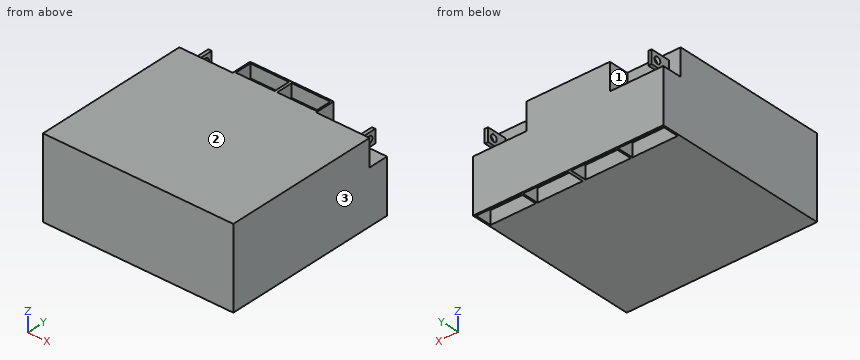
Autodesk Inventor part; units mm, degrees
ref_plane "YZ Plane" through (0, 0, 0) normal (1, 0, 0) x (0, 1, 0)
ref_plane "XZ Plane" through (0, 0, 0) normal (0, 1, 0) x (-1, 0, 0)
ref_plane "XY Plane" through (0, 0, 0) normal (0, 0, 1) x (1, 0, 0)
sketch "Sketch1" plane through (0, 0, 0) normal (0, 1, 0) x (-1, 0, 0)
  line L0 (0, 0) -> (-180.975, 0)
  line L1 (-180.975, 0) -> (-180.975, -76.2)
  line L2 (-180.975, -76.2) -> (0, -76.2)
  line L3 (0, -76.2) -> (0, 0)
  dimension "d0" = 180.975
  dimension "d1" = 76.2
extrude "Extrusion1" add sketch "Sketch1" along normal blind 168.275
sketch "Sketch2" plane through (0, 168.275, 0) normal (0, 1, 0) x (1, 0, 0)
  line L0 (0, 0) -> (180.975, 0)
  line L1 (180.975, 0) -> (180.975, 76.2)
  line L2 (180.975, 76.2) -> (0, 76.2)
  line L3 (0, 76.2) -> (0, 0)
  line L4 (0, 0) -> (50.8, 0)
  line L5 (50.8, 0) -> (50.8, 25.4)
  line L6 (50.8, 25.4) -> (0, 25.4)
  line L7 (0, 25.4) -> (0, 0)
  line L8 (180.975, 0) -> (130.175, 0)
  line L9 (130.175, 0) -> (130.175, 25.4)
  line L10 (130.175, 25.4) -> (180.975, 25.4)
  line L11 (180.975, 25.4) -> (180.975, 0)
  dimension "d4" = 50.8
  dimension "d5" = 25.4
  dimension "d6" = 50.8
  dimension "d7" = 25.4
extrude "Extrusion2" cut sketch "Sketch2" against normal blind 19.05 contours L3 L6 L5 L0 | L9 L10 L1 L0
sketch "Sketch3" plane through (0, 0, 0) normal (0, 0, 1) x (1, 0, 0)
  line L0 (50.8, 168.275) -> (50.8, 149.225) construction
  line L1 (50.8, 149.225) -> (0, 149.225)
  line L2 (0, 0) -> (0, 149.225)
  line L3 (0, 0) -> (180.975, 0)
  line L4 (180.975, 0) -> (180.975, 149.225)
  line L5 (180.975, 149.225) -> (130.175, 149.225)
  line L6 (130.175, 149.225) -> (130.175, 168.275) construction
  line L7 (50.8, 168.275) -> (130.175, 168.275) construction
  line L8 (50.8, 168.275) -> (130.175, 168.275)
  line L9 (130.175, 168.275) -> (130.175, 149.225)
  line L10 (130.175, 149.225) -> (50.8, 149.225) construction
  line L11 (50.8, 149.225) -> (50.8, 168.275)
  line L12 (52.3875, 150.8125) -> (128.5875, 150.8125) construction
  line L13 (128.5875, 150.8125) -> (128.5875, 166.6875) construction
  line L14 (128.5875, 166.6875) -> (52.3875, 166.6875) construction
  line L15 (52.3875, 166.6875) -> (52.3875, 150.8125) construction
  line L16 (52.3875, 166.6875) -> (89.2175, 166.6875)
  line L17 (89.2175, 166.6875) -> (89.2175, 150.8125)
  line L18 (89.2175, 150.8125) -> (52.3875, 150.8125)
  line L19 (52.3875, 150.8125) -> (52.3875, 166.6875)
  line L20 (128.5875, 150.8125) -> (91.7575, 150.8125)
  line L21 (91.7575, 150.8125) -> (91.7575, 166.6875)
  line L22 (91.7575, 166.6875) -> (128.5875, 166.6875)
  line L23 (128.5875, 166.6875) -> (128.5875, 150.8125)
  dimension "d10" = 1.5875
  dimension "d11" = 36.83
  dimension "d12" = 36.83
extrude "Extrusion3" cut sketch "Sketch3" against normal blind 12.7 contours L16 L17 L18 L19 | L20 L21 L22 L23
sketch "Sketch4" plane through (180.975, 0, -76.2) normal (0, 0, -1) x (-1, 0, 0)
  line L0 (0, 0) -> (180.975, 0) construction
  line L1 (180.975, 0) -> (180.975, 168.275) construction
  line L2 (0, 168.275) -> (180.975, 168.275) construction
  line L3 (0, 0) -> (0, 168.275) construction
  line L4 (0, 168.275) -> (180.975, 168.275) construction
  line L5 (180.975, 168.275) -> (180.975, 149.225) construction
  line L6 (180.975, 149.225) -> (0, 149.225) construction
  line L7 (0, 149.225) -> (0, 168.275) construction
  line L8 (1.5875, 150.8125) -> (179.3875, 150.8125) construction
  line L9 (179.3875, 150.8125) -> (179.3875, 166.6875) construction
  line L10 (179.3875, 166.6875) -> (1.5875, 166.6875) construction
  line L11 (1.5875, 166.6875) -> (1.5875, 150.8125) construction
  line L12 (1.5875, 166.6875) -> (44.5135, 166.6875)
  line L13 (44.5135, 166.6875) -> (44.5135, 150.8125)
  line L14 (44.5135, 150.8125) -> (1.5875, 150.8125)
  line L15 (1.5875, 150.8125) -> (1.5875, 166.6875)
  line L16 (179.3875, 150.8125) -> (136.4615, 150.8125)
  line L17 (136.4615, 150.8125) -> (136.4615, 166.6875)
  line L18 (136.4615, 166.6875) -> (179.3875, 166.6875)
  line L19 (179.3875, 166.6875) -> (179.3875, 150.8125)
  line L20 (46.101, 150.8125) -> (89.027, 150.8125)
  line L21 (89.027, 150.8125) -> (89.027, 166.6875)
  line L22 (89.027, 166.6875) -> (46.101, 166.6875)
  line L23 (46.101, 166.6875) -> (46.101, 150.8125)
  line L24 (134.874, 150.8125) -> (91.948, 150.8125)
  line L25 (91.948, 150.8125) -> (91.948, 166.6875)
  line L26 (91.948, 166.6875) -> (134.874, 166.6875)
  line L27 (134.874, 166.6875) -> (134.874, 150.8125)
  dimension "d15" = 1.5875
  dimension "d16" = 42.926
  dimension "d17" = 42.926
  dimension "d18" = 42.926
  dimension "d19" = 42.926
  dimension "d20" = 1.5875
  dimension "d21" = 1.5875
extrude "Extrusion4" cut sketch "Sketch4" against normal blind 12.7
sketch "Sketch5" plane through (0, 149.225, 0) normal (0, 1, 0) x (1, 0, 0)
  line L0 (50.8, 0) -> (0, 0)
  line L1 (50.8, 25.4) -> (50.8, 0)
  line L2 (0, 25.4) -> (50.8, 25.4)
  line L3 (0, 0) -> (0, 25.4)
  line L4 (180.975, 25.4) -> (180.975, 0)
  line L5 (130.175, 25.4) -> (180.975, 25.4)
  line L6 (130.175, 0) -> (130.175, 25.4)
  line L7 (180.975, 0) -> (130.175, 0)
  line L8 (0, 0) -> (12.7, 0) construction
  line L9 (12.7, 0) -> (12.7, 12.7) construction
  line L10 (12.7, 12.7) -> (0, 12.7) construction
  line L11 (0, 12.7) -> (0, 0) construction
  line L12 (180.975, 0) -> (168.275, 0) construction
  line L13 (168.275, 0) -> (168.275, 12.7) construction
  line L14 (168.275, 12.7) -> (180.975, 12.7) construction
  line L15 (180.975, 12.7) -> (180.975, 0) construction
  line L16 (11.1125, 19.05) -> (14.2875, 19.05)
  line L17 (14.2875, 19.05) -> (14.2875, 6.35)
  line L18 (14.2875, 6.35) -> (11.1125, 6.35)
  line L19 (11.1125, 6.35) -> (11.1125, 19.05)
  line L20 (11.1125, 19.05) -> (14.2875, 6.35) construction
  line L21 (14.2875, 19.05) -> (11.1125, 6.35) construction
  line L22 (169.8625, 6.35) -> (166.6875, 6.35)
  line L23 (166.6875, 6.35) -> (166.6875, 19.05)
  line L24 (166.6875, 19.05) -> (169.8625, 19.05)
  line L25 (169.8625, 19.05) -> (169.8625, 6.35)
  line L26 (169.8625, 6.35) -> (166.6875, 19.05) construction
  line L27 (166.6875, 6.35) -> (169.8625, 19.05) construction
  dimension "d24" = 12.7
  dimension "d25" = 12.7
  dimension "d26" = 12.7
  dimension "d27" = 12.7
  dimension "d28" = 3.175
  dimension "d29" = 12.7
  dimension "d30" = 3.175
  dimension "d31" = 12.7
extrude "Extrusion5" add sketch "Sketch5" along normal blind 19.05 contours L16 L17 L18 L19 | L22 L23 L24 L25
sketch "Sketch6" plane through (169.8625, 149.225, -6.35) normal (1, 0, 0) x (0, 0, -1)
  line L0 (12.7, 0) -> (0, 0) construction
  line L1 (12.7, 0) -> (12.7, 19.05) construction
  line L2 (0, 19.05) -> (12.7, 19.05) construction
  line L3 (0, 0) -> (0, 19.05) construction
  line L4 (0, 19.05) -> (6.35, 19.05) construction
  line L5 (6.35, 19.05) -> (6.35, 12.7) construction
  line L6 (6.35, 12.7) -> (0, 12.7) construction
  line L7 (0, 12.7) -> (0, 19.05) construction
  circle A0 centre (6.35, 12.7) radius 3.175
  point P0 (-6.35, -149.225)
  dimension "d34" = 6.35
  dimension "d35" = 6.35
  dimension "d36" = 6.35
extrude "Extrusion6" cut sketch "Sketch6" against normal blind 25.4
sketch "Sketch7" plane through (11.1125, 149.225, -19.05) normal (-1, 0, 0) x (0, 0, 1)
  line L0 (12.7, 0) -> (0, 0) construction
  line L1 (12.7, 0) -> (12.7, 19.05) construction
  line L2 (0, 19.05) -> (12.7, 19.05) construction
  line L3 (0, 0) -> (0, 19.05) construction
  line L4 (12.7, 19.05) -> (6.35, 19.05) construction
  line L5 (6.35, 19.05) -> (6.35, 12.7) construction
  line L6 (6.35, 12.7) -> (12.7, 12.7) construction
  line L7 (12.7, 12.7) -> (12.7, 19.05) construction
  circle A0 centre (6.35, 12.7) radius 3.175
  point P0 (19.05, -149.225)
  dimension "d39" = 6.35
  dimension "d40" = 6.35
  dimension "d41" = 6.35
extrude "Extrusion7" cut sketch "Sketch7" against normal blind 25.4
properties part number "battery"
Verification items for the finished model (mm, model axes). Face numbers are marked on the shaded views. Coordinates: 2 decimals unless noted, no trailing zeros. Loops run counter-clockwise (first coordinate to the right, second up) from the corner with the lowest first, then second, coordinate; pieces in that order, holes last. Notation, with made-up numbers: (15, 15) -> (38, 15) arc R8 cw to (38, 26) -> close; hole circle Ø5 at (73.5, 58.5). An arc over 180 degrees is marked (long way). Answer as a JSON object with one key per item and string values. Group by question number.
Item 1: Mould release check, pull along X, two halves, no side actions. Record for the marked faces 1, 2 and 3: +X half, -X half, draft (parallel to the pull), parting line (faces both ways), or undercut.
Item 2: Sectioned sample at A-A on x = 56. Record the boundary of the cut face in (y, z) (1 decimal), plus the area to 3 significant figures.
Item 3: Depth check by flat-ended pin: pin 1 (5.5 mm diameter, centred on y = 158.5, z = -18.5, fed in from +X); pin 2 (9.5 mm diameter, centred on y = 163, z = -11, fed in from -X). Enter the tip coordinate at first touch or a pass-through.
Item 4: Scan lines: probe 1 along Y at (x, z) = (13.1, -12.7) (3 decimals); probe 2 along Y at (x, z) = (118.5, -73) (1 decimal); probe 3 along Y at (x, z) = (22, -19) (3 decimals). Record each from-to range of solid material in increasing order.
Evaluation:
{
 "1": {"face 1": "undercut", "face 2": "draft", "face 3": "+X half"},
 "2": {"outline": "(0, -76.2) -> (150.8, -76.2) -> (150.8, -63.5) -> (166.7, -63.5) -> (166.7, -76.2) -> (168.3, -76.2) -> (168.3, 0) -> (166.7, 0) -> (166.7, -12.7) -> (150.8, -12.7) -> (150.8, 0) -> (0, 0) -> close", "area": "12,400 mm²"},
 "3": {"pin 1": "stops at x = 169.86", "pin 2": "stops at x = 11.11"},
 "4": {"probe 1": "y = 0 to 158.75, 165.1 to 168.275", "probe 2": "y = 0 to 150.8, 166.7 to 168.3", "probe 3": "y = 0 to 149.225"}
}
